Input: part model. Units: mm. Frame: model coordinates. Face numbers are marked on the shaded views. A direction names the side the tool comes from. Give positions to 0.01 mm unless a question says otherwise; leave off trailing zeros. Order: outer loops, then holes, each group sorted by start corner. A loop starts at its lowest first (then second) coordinate and runs counter-clockwise, first axis right, second up. Notation, with made-up numbers: M 88.25,-38 L 131.25,-38 A25 cw 131.25,-2 Z; hole C 81.5,48.5 d8. An arc over 180 degrees is marked long. Use a Markdown table: item, result.
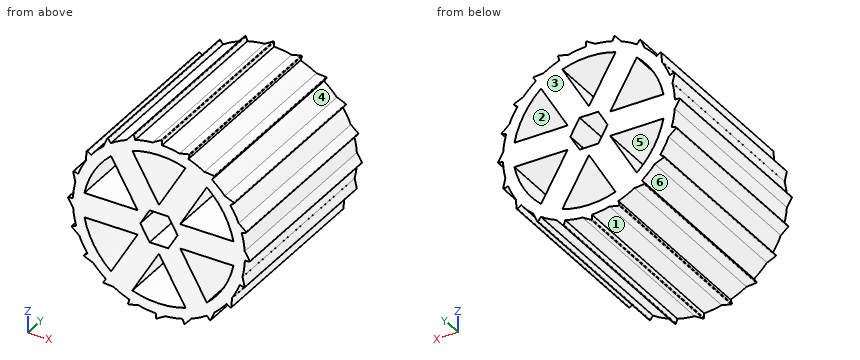
from build123d import *

# Parameters (mm, degrees)
SKETCH1_R           = 35.56
BOSS_EXTRUDE1_DEPTH = 76.2
CUT_EXTRUDE1_DEPTH  = 76.2
CUT_EXTRUDE2_DEPTH  = 76.2
BOSS_EXTRUDE2_DEPTH = 76.2
FILLET1_R           = 0.254


with BuildPart() as part:
    # Sketch1 → Boss-Extrude1 (new body)
    with BuildSketch(Plane(origin=(0, 0, 0), x_dir=(1, 0, 0), z_dir=(0, 1, 0))):
        with Locations(Location((0, 0, 0), (0, 0, 90))):
            Circle(SKETCH1_R)
    extrude(amount=BOSS_EXTRUDE1_DEPTH)

    # Sketch2 → Cut-Extrude1 (cut)
    with BuildSketch(Plane(origin=(0, 76.2, 0), x_dir=(1, 0, 0), z_dir=(0, 1, 0))):
        Polygon((7.69896584, 0), (3.84948292, 6.6675), (-3.84948292, 6.6675), (-7.69896584, 0), (-3.84948292, -6.6675), (3.84948292, -6.6675), align=None)
    extrude(amount=-CUT_EXTRUDE1_DEPTH, mode=Mode.SUBTRACT)

    # Sketch3 → Cut-Extrude2 (cut)
    with BuildSketch(Plane(origin=(0, 76.2, 0), x_dir=(1, 0, 0), z_dir=(0, 1, 0))):
        with BuildLine():
            Line((8.798818102, 5.08), (30.795863359, 5.08))
            ThreePointArc((30.795863359, 5.08), (26.854956532, 15.504716383), (19.797340731, 24.13))
            Line((19.797340731, 24.13), (8.798818102, 5.08))
        make_face()
        with BuildLine():
            Line((0, 10.16), (10.998522628, 29.21))
            ThreePointArc((10.998522628, 29.21), (0, 31.009432765), (-10.998522628, 29.21))
            Line((-10.998522628, 29.21), (0, 10.16))
        make_face()
        with BuildLine():
            Line((8.798818102, -5.08), (19.797340731, -24.13))
            ThreePointArc((19.797340731, -24.13), (26.854956532, -15.504716383), (30.795863359, -5.08))
            Line((30.795863359, -5.08), (8.798818102, -5.08))
        make_face()
        with BuildLine():
            Line((0, -10.16), (-10.998522628, -29.21))
            ThreePointArc((-10.998522628, -29.21), (0, -31.009432765), (10.998522628, -29.21))
            Line((10.998522628, -29.21), (0, -10.16))
        make_face()
        with BuildLine():
            Line((-8.798818102, -5.08), (-30.795863359, -5.08))
            ThreePointArc((-30.795863359, -5.08), (-26.854956532, -15.504716383), (-19.797340731, -24.13))
            Line((-19.797340731, -24.13), (-8.798818102, -5.08))
        make_face()
        with BuildLine():
            Line((-8.798818102, 5.08), (-19.797340731, 24.13))
            ThreePointArc((-19.797340731, 24.13), (-26.854956532, 15.504716383), (-30.795863359, 5.08))
            Line((-30.795863359, 5.08), (-8.798818102, 5.08))
        make_face()
    extrude(amount=-CUT_EXTRUDE2_DEPTH, mode=Mode.SUBTRACT)

    # Sketch4 → Boss-Extrude2 (add)
    with BuildSketch(Plane(origin=(0, 76.2, 0), x_dir=(1, 0, 0), z_dir=(0, 1, 0))):
        Polygon((10.506917468, 36.313470126), (9.069726639, 32.155431824), (13.389288853, 32.989807207), align=None)
        Polygon((2.539559344, 35.512688914), (-1.22880707, 37.782978449), (-1.310752274, 33.384332637), align=None)
        Polygon((21.214151718, 31.289346337), (18.562397516, 27.778933305), (22.92838148, 27.237653318), align=None)
        Polygon((29.84479699, 23.202403322), (26.238051593, 20.683239247), (30.223084377, 18.819288146), align=None)
        Polygon((35.554025592, 12.84424741), (31.345342368, 11.562925622), (34.559341198, 8.558759928), align=None)
        Polygon((37.782978449, 1.22880707), (33.384332637, 1.310752274), (35.512688914, -2.539559344), align=None)
        Polygon((36.313470126, -10.506917468), (32.155431824, -9.069726639), (32.989807207, -13.389288853), align=None)
        Polygon((31.289346337, -21.214151718), (27.778933305, -18.562397516), (27.237653318, -22.92838148), align=None)
        Polygon((23.202403322, -29.84479699), (20.683239247, -26.238051593), (18.819288146, -30.223084377), align=None)
        Polygon((12.84424741, -35.554025592), (11.562925622, -31.345342368), (8.558759928, -34.559341198), align=None)
        Polygon((1.22880707, -37.782978449), (1.310752274, -33.384332637), (-2.539559344, -35.512688914), align=None)
        Polygon((-10.506917468, -36.313470126), (-9.069726639, -32.155431824), (-13.389288853, -32.989807207), align=None)
        Polygon((-21.214151718, -31.289346337), (-18.562397516, -27.778933305), (-22.92838148, -27.237653318), align=None)
        Polygon((-29.84479699, -23.202403322), (-26.238051593, -20.683239247), (-30.223084377, -18.819288146), align=None)
        Polygon((-35.554025592, -12.84424741), (-31.345342368, -11.562925622), (-34.559341198, -8.558759928), align=None)
        Polygon((-37.782978449, -1.22880707), (-33.384332637, -1.310752274), (-35.512688914, 2.539559344), align=None)
        Polygon((-36.313470126, 10.506917468), (-32.155431824, 9.069726639), (-32.989807207, 13.389288853), align=None)
        Polygon((-31.289346337, 21.214151718), (-27.778933305, 18.562397516), (-27.237653318, 22.92838148), align=None)
        Polygon((-23.202403322, 29.84479699), (-20.683239247, 26.238051593), (-18.819288146, 30.223084377), align=None)
        Polygon((-12.84424741, 35.554025592), (-11.562925622, 31.345342368), (-8.558759928, 34.559341198), align=None)
    extrude(amount=-BOSS_EXTRUDE2_DEPTH)

    # Fillet1
    fillet1_edges = [part.edges().sort_by_distance(p)[0] for p in [
        (-1.22880707, 38.1, -37.782978449),
        (10.506917468, 38.1, -36.313470126),
        (21.214151718, 38.1, -31.289346337),
        (29.84479699, 38.1, -23.202403322),
        (35.554025592, 38.1, -12.84424741),
        (37.782978449, 38.1, -1.22880707),
        (36.313470126, 38.1, 10.506917468),
        (31.289346337, 38.1, 21.214151718),
        (23.202403322, 38.1, 29.84479699),
        (12.84424741, 38.1, 35.554025592),
        (1.22880707, 38.1, 37.782978449),
        (-10.506917468, 38.1, 36.313470126),
        (-21.214151718, 38.1, 31.289346337),
        (-29.84479699, 38.1, 23.202403322),
        (-35.554025592, 38.1, 12.84424741),
        (-37.782978449, 38.1, 1.22880707),
        (-36.313470126, 38.1, -10.506917468),
        (-31.289346337, 38.1, -21.214151718),
        (-23.202403322, 38.1, -29.84479699),
        (-12.84424741, 38.1, -35.554025592),
    ]]
    fillet(fillet1_edges, radius=FILLET1_R)


solid = part.part
1) Cut plane C-C on y = 10. State how many separate pieces and enclosed holes the cut face has, and give its area (3 significant figures).
Response values:
| item | result |
|---|---|
| separate pieces | 1 |
| enclosed holes | 7 |
| area | 2,490 mm² |
2) Mould query, pull axis Z, two halves, no side actions, for the marked faces 1, 2 and 3. Classes: released by +Z, released by -Z, zero draft, split by the parting line, or undercut.
Response values:
| item | result |
|---|---|
| face 1 | released by -Z |
| face 2 | undercut |
| face 3 | zero draft |
3) Cut plane B-B on x = 26. Return loops of the section in (y, z), and give its area (3 significant figures).
Response values:
| item | result |
|---|---|
| outline | M 0,-24.26 L 76.2,-24.26 L 76.2,-16.91 L 0,-16.91 Z; M 0,-5.08 L 76.2,-5.08 L 76.2,5.08 L 0,5.08 Z; M 0,16.91 L 76.2,16.91 L 76.2,24.26 L 0,24.26 Z |
| area | 1,890 mm² |
4) First-contact query: pin 1 Ø10 at (x, y) = (27, 11.5) entering from -Z; pin 2 Ø6.5 at (x, y) = (-23.5, 48.5) entering from +Z; pin 3 Ø8 at (x, z) = (-16.5, -6) entering from -Y; pin 4 Ø17.5 at (x, y) = (-20.5, 22) entering from -Z. Flat tips, straight axial feed; report the tip coordinate or a pass-through.
Response values:
| item | result |
|---|---|
| pin 1 | stops at z = -29.43 |
| pin 2 | stops at z = 31.04 |
| pin 3 | stops at y = 0 |
| pin 4 | stops at z = -35.46 |
5) Material intervals for line 1 (X direction, y = 46.5, z = -18); line 2 (Z direction, x = -24, y = 32); line 3 (Z direction, x = 15.5, y = 51), sorted ascending. Write a range as from..to.
Response values:
| item | result |
|---|---|
| line 1 | x = -30.67..-25.27, -16.26..-4.53, 4.53..16.26, 25.27..30.67 |
| line 2 | z = -26.24..-19.7, -5.08..5.08, 19.7..26.24 |
| line 3 | z = -32..-16.69, -5.08..5.08, 16.69..32 |
6) Cut plane A-A on z = -17. Return loops of the section in (x, y).
Response values:
| item | result |
|---|---|
| outline | M -31.23,0 L -25.94,0 L -25.94,76.2 L -31.23,76.2 Z; M -15.68,0 L -3.95,0 L -3.95,76.2 L -15.68,76.2 Z; M 3.95,0 L 15.68,0 L 15.68,76.2 L 3.95,76.2 Z; M 25.94,0 L 31.23,0 L 31.23,76.2 L 25.94,76.2 Z |
7) Reachability of the marked faces 4, 5 and 6 from +Z, -Z, +X, -X, +Y, -Y: full face, straight path, thin tool, end or side. Return the list, or none.
Response values:
| item | result |
|---|---|
| face 4 | +X, +Y, -Y |
| face 5 | +Y, -Y |
| face 6 | -X, +Y, -Y |
